from build123d import *

# Parameters (mm, degrees)
SKETCH1_R           = 5
BOSS_EXTRUDE1_DEPTH = 6
SKETCH2_R           = 1.3
CUT_EXTRUDE1_DEPTH  = 256.119579805
LPATTERN1_COUNT     = 10
LPATTERN1_PITCH     = 25
CUT_EXTRUDE3_DEPTH  = 256.119579805
BOSS_EXTRUDE2_DEPTH = 6
CUT_EXTRUDE4_DEPTH  = 257.947465448
BOSS_EXTRUDE3_DEPTH = 6


with BuildPart() as part:
    # Sketch1 → Boss-Extrude1 (new body)
    with BuildSketch(Plane.XY):
        with BuildLine():
            Line((250, 5), (0, 5))
            ThreePointArc((0, 5), (3.535533906, 3.535533906), (5, 0))
            ThreePointArc((5, 0), (3.535533906, -3.535533906), (0, -5))
            Line((0, -5), (250, -5))
            ThreePointArc((250, -5), (245, 0), (250, 5))
        make_face()
        with Locations((250, 0)):
            Circle(SKETCH1_R)
        Circle(SKETCH1_R)
    extrude(amount=BOSS_EXTRUDE1_DEPTH)

    # Sketch2 → Cut-Extrude1 (cut, through all)
    with BuildSketch(Plane.XY.offset(6)):
        Circle(SKETCH2_R)
        with Locations((250, 0)):
            Circle(SKETCH2_R)
    cut_extrude1 = extrude(amount=-CUT_EXTRUDE1_DEPTH, mode=Mode.SUBTRACT)

    # LPattern1: Cut-Extrude1 ×10
    with Locations(*[(i * LPATTERN1_PITCH, 0, 0) for i in range(1, LPATTERN1_COUNT)]):
        add(cut_extrude1, mode=Mode.SUBTRACT)

    # Sketch3 → Cut-Extrude3 (cut, through all)
    with BuildSketch(Plane.XY.offset(6)):
        with BuildLine():
            ThreePointArc((250, -1.3), (248.874166975, 0.65), (251.125833025, 0.65))
            Line((251.125833025, 0.65), (248.614359354, 5))
            Line((248.614359354, 5), (236.796717724, 5))
            Line((236.796717724, 5), (238.778399593, -0.444626186))
            ThreePointArc((238.778399593, -0.444626186), (239.254350633, -1.064897658), (240, -1.3))
            Line((240, -1.3), (250, -1.3))
        make_face()
    extrude(amount=-CUT_EXTRUDE3_DEPTH, mode=Mode.SUBTRACT)

    # Sketch3<4> → Boss-Extrude2 (add, through all)
    with BuildSketch(Plane.XY.offset(6)):
        with BuildLine():
            Line((216.469850466, 5), (236.796717724, 5))
            Line((236.796717724, 5), (227.572976716, 30.342020143))
            ThreePointArc((227.572976716, 30.342020143), (226.633284095, 31), (225.693591475, 30.342020143))
            Line((225.693591475, 30.342020143), (216.469850466, 5))
        make_face()
    extrude(amount=-BOSS_EXTRUDE2_DEPTH)

    # Sketch4 → Cut-Extrude4 (cut, through all)
    with BuildSketch(Plane.XY.offset(6)):
        with BuildLine():
            Line((225.411683688, 17.872267266), (221.361553558, 6.744626186))
            ThreePointArc((221.361553558, 6.744626186), (221.518256307, 5.554350633), (222.583153965, 5))
            Line((222.583153965, 5), (230.683414226, 5))
            ThreePointArc((230.683414226, 5), (231.748311883, 5.554350633), (231.905014633, 6.744626186))
            Line((231.905014633, 6.744626186), (227.854884502, 17.872267266))
            ThreePointArc((227.854884502, 17.872267266), (226.633284095, 18.727641079), (225.411683688, 17.872267266))
        make_face()
    extrude(amount=-CUT_EXTRUDE4_DEPTH, mode=Mode.SUBTRACT)

    # Sketch5 → Boss-Extrude3 (add, through all)
    with BuildSketch(Plane.XY.offset(6)):
        with BuildLine():
            ThreePointArc((110.857864376, 5), (115.8563971, 11.890943024), (123.8, 14.951922953))
            Line((123.8, 14.951922953), (-0.4, 4.983974318))
            ThreePointArc((-0.4, 4.983974318), (-0.20016045, 4.995991973), (0, 5))
            Line((0, 5), (110.857864376, 5))
        make_face()
        with BuildLine():
            ThreePointArc((0, -5), (-0.20016045, -4.995991973), (-0.4, -4.983974318))
            Line((-0.4, -4.983974318), (123.8, -14.951922953))
            ThreePointArc((123.8, -14.951922953), (115.8563971, -11.890943024), (110.857864376, -5))
            Line((110.857864376, -5), (0, -5))
        make_face()
        with BuildLine():
            ThreePointArc((125.982164337, 14.967810568), (124.890792866, 14.999602455), (123.8, 14.951922953))
            ThreePointArc((123.8, 14.951922953), (115.8563971, 11.890943024), (110.857864376, 5))
            Line((110.857864376, 5), (139.142135624, 5))
            ThreePointArc((139.142135624, 5), (134.056788847, 11.957197656), (125.982164337, 14.967810568))
        make_face()
        with BuildLine():
            Line((139.142135624, -5), (110.857864376, -5))
            ThreePointArc((110.857864376, -5), (115.8563971, -11.890943024), (123.8, -14.951922953))
            ThreePointArc((123.8, -14.951922953), (125, -15), (126.2, -14.951922953))
            ThreePointArc((126.2, -14.951922953), (134.1436029, -11.890943024), (139.142135624, -5))
        make_face()
        with BuildLine():
            Line((250, -5), (139.142135624, -5))
            ThreePointArc((139.142135624, -5), (134.1436029, -11.890943024), (126.2, -14.951922953))
            Line((126.2, -14.951922953), (250.4, -4.983974318))
            ThreePointArc((250.4, -4.983974318), (250.20016045, -4.995991973), (250, -5))
        make_face()
        with BuildLine():
            Line((216.929325308, 9), (125.982164337, 14.967810568))
            ThreePointArc((125.982164337, 14.967810568), (134.056788847, 11.957197656), (139.142135624, 5))
            Line((139.142135624, 5), (216.469850466, 5))
            Line((216.469850466, 5), (218.236046624, 9.852584063))
            ThreePointArc((218.236046624, 9.852584063), (217.724813241, 9.208459271), (216.929325308, 9))
        make_face()
        with BuildLine():
            Line((240, -1.3), (250, -1.3))
            Line((250, -1.3), (239.61442594, -0.50835284))
            ThreePointArc((239.61442594, -0.50835284), (238.927624535, -0.247883379), (238.491632246, 0.343260625))
            Line((238.491632246, 0.343260625), (238.778399593, -0.444626186))
            ThreePointArc((238.778399593, -0.444626186), (239.254350633, -1.064897658), (240, -1.3))
        make_face()
    extrude(amount=-BOSS_EXTRUDE3_DEPTH)


solid = part.part
Here's how the part is built. I have some questions about the finished solid (model axes, mm). A direction names the side the tool comes from. Coordinates: 2 decimals unless noted, no trailing zeros. Order: outer loops, then holes, each group sorted by start corner. A loop starts at its lowest first (then second) coordinate and runs counter-clockwise, first axis right, second up.
Item 1: If we section it at C-C on x = 42: List the corners of the cut face in (y, z) for me.
Result sheet:
outline: (-8.39, 0) - (8.39, 0) - (8.39, 6) - (-8.39, 6) - close
Item 2: For P1, Ø1.5, axis at x = 249.5, z = 4, coming from the +Y side, with a flat end and sliding along its axis, tell me the tip position at first contact or that it passes through.
Result sheet:
P1: stops at y = 5
Item 3: If we mould it in two halves opening along Y, with no side actions, what happens to faces 4 (the face through (123, -2, 6)), 5 (the face through (60.83, -9.9, 3.04)), 6 (the face through (227, 5, 3))? For each: +Y half, -Y half, draft (parallel to the pull), parting line (faces both ways), or undercut.
Result sheet:
face 4: draft
face 5: -Y half
face 6: undercut
Item 4: If we section it at A-A on z = 2.25: State how many separate pieces and enclosed holes the cut face has, plus the area to 3 significant figures.
Result sheet:
separate pieces: 1
enclosed holes: 11
area: 5,180 mm2
Item 5: I need wall thicknesses on line 1 (Y direction, x = 125, z = 2.05); line 2 (X direction, y = 18.5, z = 2.5); line 3 (X direction, y = 16.5, z = 5). Which ranges of each line are inside material? Lowest first, please.
Result sheet:
line 1: y = -15 to -1.3, 1.3 to 15
line 2: x = 221.38 to 225.9, 227.37 to 231.88
line 3: x = 220.66 to 224.91, 228.35 to 232.61
Item 6: If we section it at B-B on y = 12: List the corners of the cut face in (x, z) for me.
Result sheet:
outline: (87.02, 0) - (171.21, 0) - (171.21, 6) - (87.02, 6) - close; (219.02, 0) - (223.27, 0) - (223.27, 6) - (219.02, 6) - close; (229.99, 0) - (234.25, 0) - (234.25, 6) - (229.99, 6) - close
Item 7: For faces 1 (the face through (249.89, 2.79, 3.04)), 2 (the face through (222.017, 20.241, 3.042)), 3 (the face through (123, -2, 0)), which set-ups out of +Z, -Z, +X, -X, +Y, -Y let a thin tool reach every point of the face, with its end or its side?
Result sheet:
face 1: +Z, -Z
face 2: +Z, -Z, +Y
face 3: -Z, +X, -X, +Y, -Y
